```python
from build123d import *

# Parameters (mm, degrees)
EXTRUDE_1_DEPTH   = 5
EXTRUDE_1_2_DEPTH = 5


# Read off the part's stored shape, not the designer's step: 拉伸-薄壁1
with BuildPart() as part:
    # Extrude 1 outline → Extrude 1 (new body)
    with BuildSketch(Plane.XY):
        with BuildLine():
            ThreePointArc((-91.999999998, -43.29999887), (-91.998341789, -43.340687344), (-91.993377975, -43.381105931))
            Line((-91.993377975, -43.381105931), (-81.999999998, -43.29999887))
            Line((-81.999999998, -43.29999887), (-81.999999998, -41.231306411))
            ThreePointArc((-81.999999998, -41.231306411), (-68.990237418, -27.264516088), (-65.018315032, -8.595049387))
            Line((-65.018315032, -8.595049387), (-66.717183167, 19.436274835))
            Line((-66.717183167, 19.436274835), (-41.506651541, 41))
            Line((-41.506651541, 41), (41.506651544, 41))
            Line((41.506651544, 41), (66.717183171, 19.436274835))
            Line((66.717183171, 19.436274835), (65.018315035, -8.595049396))
            ThreePointArc((65.018315035, -8.595049396), (68.990237423, -27.264516092), (82.000000002, -41.231306411))
            Line((82.000000002, -41.231306411), (82.000000002, -57.596758434))
            Line((82.000000002, -57.596758434), (69.128212183, -137.203815401))
            ThreePointArc((69.128212183, -137.203815401), (66.269370107, -168.113208397), (67.632339208, -199.124591285))
            Line((67.632339208, -199.124591285), (57.095329321, -203.866245712))
            Line((57.095329321, -203.866245712), (2e-09, -195.082348893))
            Line((2e-09, -195.082348893), (-57.095329308, -203.86624571))
            Line((-57.095329308, -203.86624571), (-67.632339202, -199.124591258))
            ThreePointArc((-67.632339202, -199.124591258), (-66.269370105, -168.113208363), (-69.128212188, -137.20381536))
            Line((-69.128212188, -137.20381536), (-81.999822911, -57.597853653))
            Line((-81.999822911, -57.597853653), (-81.996689231, -43.383854869))
            Line((-81.996689231, -43.383854869), (-91.996688988, -43.381650225))
            Line((-91.996688988, -43.381650225), (-91.999999999, -58.4))
            Line((-91.999999999, -58.4), (-79.000000006, -138.79999996))
            ThreePointArc((-79.000000006, -138.79999996), (-76.209004677, -171.980865978), (-78.499999999, -205.199999999))
            Line((-78.499999999, -205.199999999), (-58.499999998, -214.2))
            Line((-58.499999998, -214.2), (2e-09, -205.199999999))
            Line((2e-09, -205.199999999), (58.500000002, -214.2))
            Line((58.500000002, -214.2), (78.500000007, -205.200000039))
            ThreePointArc((78.500000007, -205.200000039), (76.209004679, -171.980866018), (79.000000002, -138.799999999))
            Line((79.000000002, -138.799999999), (92.000000002, -58.4))
            Line((92.000000002, -58.4), (92.000000002, -35.349095722))
            ThreePointArc((92.000000002, -35.349095722), (91.910917667, -35.064233027), (91.675413177, -34.880875309))
            ThreePointArc((91.675413177, -34.880875309), (79.107890632, -24.786992353), (75.000000002, -9.2))
            Line((75.000000002, -9.2), (76.984943405, 23.551566159))
            ThreePointArc((76.984943405, 23.551566159), (76.946128848, 23.777138637), (76.810861071, 23.961779211))
            Line((76.810861071, 23.961779211), (45.340334501, 50.87996546))
            ThreePointArc((45.340334501, 50.87996546), (45.188562585, 50.969032371), (45.015332579, 51))
            Line((45.015332579, 51), (-45.015332561, 51))
            ThreePointArc((-45.015332561, 51), (-45.188562568, 50.969032376), (-45.340334486, 50.879965469))
            Line((-45.340334486, 50.879965469), (-76.810861028, 23.961779245))
            ThreePointArc((-76.810861028, 23.961779245), (-76.946128824, 23.777138686), (-76.984943405, 23.551566212))
            Line((-76.984943405, 23.551566212), (-74.999999999, -9.199999994))
            ThreePointArc((-74.999999999, -9.199999994), (-79.107890627, -24.786992351), (-91.675413174, -34.880875309))
            ThreePointArc((-91.675413174, -34.880875309), (-91.910917622, -35.064232967), (-91.999999998, -35.349095576))
            Line((-91.999999998, -35.349095576), (-91.999999998, -43.29999887))
        make_face()
    extrude(amount=EXTRUDE_1_DEPTH)

    # 草图7 → Extrude 1 2 (add)
    with BuildSketch(Plane.XY):
        with BuildLine():
            Line((-81.999999998, -43.29999887), (-83.629600195, -43.313224837))
            Line((-83.629600195, -43.313224837), (-83.629600195, -43.38349487))
            Line((-83.629600195, -43.38349487), (-81.996689231, -43.383854869))
            Line((-81.996689231, -43.383854869), (-81.999822911, -57.597853653))
            Line((-81.999822911, -57.597853653), (-69.128212188, -137.20381536))
            ThreePointArc((-69.128212188, -137.20381536), (-69.063707743, -137.605017492), (-68.999917919, -138.006333867))
            Line((-68.999917919, -138.006333867), (-68.990237418, -138.006333867))
            Line((-68.990237418, -138.006333867), (-68.990237418, -138.06764197))
            ThreePointArc((-68.990237418, -138.06764197), (-66.259225934, -168.550479027), (-67.632339202, -199.124591258))
            Line((-67.632339202, -199.124591258), (-57.095329308, -203.86624571))
            Line((-57.095329308, -203.86624571), (2e-09, -195.082348893))
            Line((2e-09, -195.082348893), (57.095329321, -203.866245712))
            Line((57.095329321, -203.866245712), (67.632339208, -199.124591285))
            ThreePointArc((67.632339208, -199.124591285), (66.269370107, -168.113208397), (69.128212183, -137.203815401))
            Line((69.128212183, -137.203815401), (82.000000002, -57.596758434))
            Line((82.000000002, -57.596758434), (82.000000002, -41.231306411))
            ThreePointArc((82.000000002, -41.231306411), (68.990237423, -27.264516092), (65.018315035, -8.595049396))
            Line((65.018315035, -8.595049396), (66.717183171, 19.436274835))
            Line((66.717183171, 19.436274835), (41.506651544, 41))
            Line((41.506651544, 41), (-41.506651541, 41))
            Line((-41.506651541, 41), (-66.717183167, 19.436274835))
            Line((-66.717183167, 19.436274835), (-65.018315032, -8.595049387))
            ThreePointArc((-65.018315032, -8.595049387), (-68.990237418, -27.264516088), (-81.999999998, -41.231306411))
            Line((-81.999999998, -41.231306411), (-81.999999998, -43.29999887))
        make_face()
    extrude(amount=EXTRUDE_1_2_DEPTH)


solid = part.part
```
Build history of the part. All positions in model axes, mm. A direction names the side the tool comes from. Give positions to 0.01 mm unless a question says otherwise; leave off trailing zeros. Loops run counter-clockwise (first coordinate to the right, second up) from the corner with the lowest first, then second, coordinate; pieces in that order, holes last. Notation, with made-up numbers: (-8.5, 12.25) - (42.5, 12.25) arc R27 cw to (42.5, 46.25) - close; hole circle Ø11 at (62, 3). An arc over 180 degrees is marked (long way). Use a Markdown table: item, result.
(1) Band-saw the part on C-C (x = 8). Give the cut face in (y, z).
Taken from the geometry:
| item | result |
|---|---|
| outline | (-206.43, 0) - (51, 0) - (51, 5) - (-206.43, 5) - close |
(2) Band-saw the part on B-B (y = 30). Give the cut face in (x, z), and give its area (3 significant figures).
Taken from the geometry:
| item | result |
|---|---|
| outline | (-69.75, 0) - (69.75, 0) - (69.75, 5) - (-69.75, 5) - close |
| area | 698 mm2 |
(3) Pull direction X, two halves, no side cores. Call faces 4 (the face through (85.41, -99.16, 2.46)), 5 (the face through (28.841, -209.637, 2.465)), 6 (the face through (-92, -39, 2)), 7 (the face through (-29.659, -209.763, 2.465)): +X half, -X half, draft (parallel to the pull), parting line (faces both ways), or undercut.
Taken from the geometry:
| item | result |
|---|---|
| face 4 | +X half |
| face 5 | undercut |
| face 6 | -X half |
| face 7 | undercut |
(4) Which spindle directions (+Z, -Z, +X, -X, +Y, -Y) get a long thin tool onto all of the face, cutting with end or side? Do faces 1 (the face through (-1, -80, 0)), 2 (the face through (79.234, -24.979, 2.465)), 3 (the face through (-76.006, 7.405, 2.465)). Say none if no direction does.
Taken from the geometry:
| item | result |
|---|---|
| face 1 | -Z, +X, -X, +Y, -Y |
| face 2 | +Z, -Z, +X |
| face 3 | +Z, -Z, -X |
(5) Drop flat-ended pins along their axis: pin 1 Ø1 at (x, y) = (45.5, -54.5) entering from -Z; pin 2 Ø1 at (y, z) = (-107, 2) entering from +X; pin 3 Ø1.5 at (x, z) = (-86.5, 3.5) entering from +Y. Give the stop position or say it passes through.
Taken from the geometry:
| item | result |
|---|---|
| pin 1 | z = 0 |
| pin 2 | x = 84.22 |
| pin 3 | y = -31.73 |
(6) Wall check: line 1 along X through (y, z) = (13, 3.95); line 2 along Y through (x, z) = (-45, 3.1); line 3 along X through (y, z) = (-4.5, 3.4). Give the ranges that are in metal, low to high.
Taken from the geometry:
| item | result |
|---|---|
| line 1 | -76.35 to 76.35 |
| line 2 | -212.12 to 51 |
| line 3 | -75.28 to 75.28 |
